Geometry check sheet. Reference: the model listing, model coordinates, mm. Coordinates: 2 decimals unless noted, no trailing zeros. Order: outer loops, then holes, each group sorted by start corner. A loop starts at its lowest first (then second) coordinate and runs counter-clockwise, first axis right, second up. Notation, with made-up numbers: M -22.5,-26.75 L 13.5,-26.75 A17 cw 13.5,-14.75 Z; hole C -37.5,5.25 d11. An arc over 180 degrees is marked long. One line per item, written item: value. Start each with the question number.
1) Go/stop test with flat-tipped pins: P1, Ø1.5, axis at y = 10, z = 2, coming from the -X side; P2, Ø1, axis at x = 6, z = 0.5, coming from the -Y side; P3, Ø2, axis at y = 12, z = -0.5, coming from the +X side. Record where each tip stops, or that it passes through.
2) Draft check along X on faces 1 (the cylindrical face through (-4.336, -19.524, 0.042)), 2 (the cylindrical face through (1.5, 0.07, -0.04)), 3 (the flat face through (4, 0, 3)). Enter one of: pulls with the +X half, pulls with the -X half, needs draft (parallel to the pull), parting line crosses it, or undercut.
3) Thickness scan on L1, parallel to Y at x = 0, z = 0.05; L2, parallel to X at y = -11, z = 0.9; L3, parallel to Y at x = -9.5, z = -0.85. Record the ranges inside material, lowest first. Write a range as from..to.
4) Sectioned sample at A-A, the plane x = 0. Enter the section's corners in (y, z).
5) Sectioned sample at C-C, the plane z = -1.8. Enter the section's corners in (x, y), then the cut area to 3 significant figures.
6) Sectioned sample at D-D, the plane y = -16. Enter the section's corners in (x, z), then the cut area to 3 significant figures.
```python
from build123d import *

# Parameters (mm, degrees)
F0_R     = 20
F1_DEPTH = 3
F2_D     = 3
F3_D     = 3


with BuildPart() as f1:
    # F0 (on Top) → F1 (new body, symmetric)
    with BuildSketch(Plane.XY):
        Circle(F0_R)
    extrude(amount=F1_DEPTH, both=True)

    # F2 (through all)
    with Locations(Plane.XY):
        with Locations((0, 0)):
            Hole(F2_D / 2)

    # F3 (through all)
    with Locations(Plane(origin=(0, 0, 0), x_dir=(1, 0, 0), z_dir=(0, 0, -1))):
        with Locations((0, 0)):
            Hole(F3_D / 2)


solid = f1.part
```
Final values:
1. P1: stops at x = -17.73
1. P2: stops at y = -19.23
1. P3: stops at x = 16.7
2. face 1: parting line crosses it
2. face 2: undercut
2. face 3: needs draft
3. L1: y = -20..-1.5, 1.5..20
3. L2: x = -16.7..16.7
3. L3: y = -17.6..17.6
4. outline: M -20,-3 L -1.5,-3 L -1.5,3 L -20,3 Z; M 1.5,-3 L 20,-3 L 20,3 L 1.5,3 Z
5. outline: C 0,0 d40; hole C 0,0 d3
5. area: 1,250 mm^2
6. outline: M -12,-3 L 12,-3 L 12,3 L -12,3 Z
6. area: 144 mm^2
